Verification items for this drawing (mm, ordinates from the low corner). A direction names the side the tool comes from. Give positions to 0.01 mm unless a question says otherwise; leave off trailing zeros. Loops run counter-clockwise (first coordinate to the right, second up) from the corner with the lowest first, then second, coordinate; pieces in that order, holes last. Notation, with made-up numbers: (53, 64.25) -> (62, 64.25) arc R24 cw to (62, 81.25) -> close; hole circle Ø11 at (-22, 64). An arc over 180 degrees is marked (long way). Use one line per item in the form item = value. Start each with the question number.
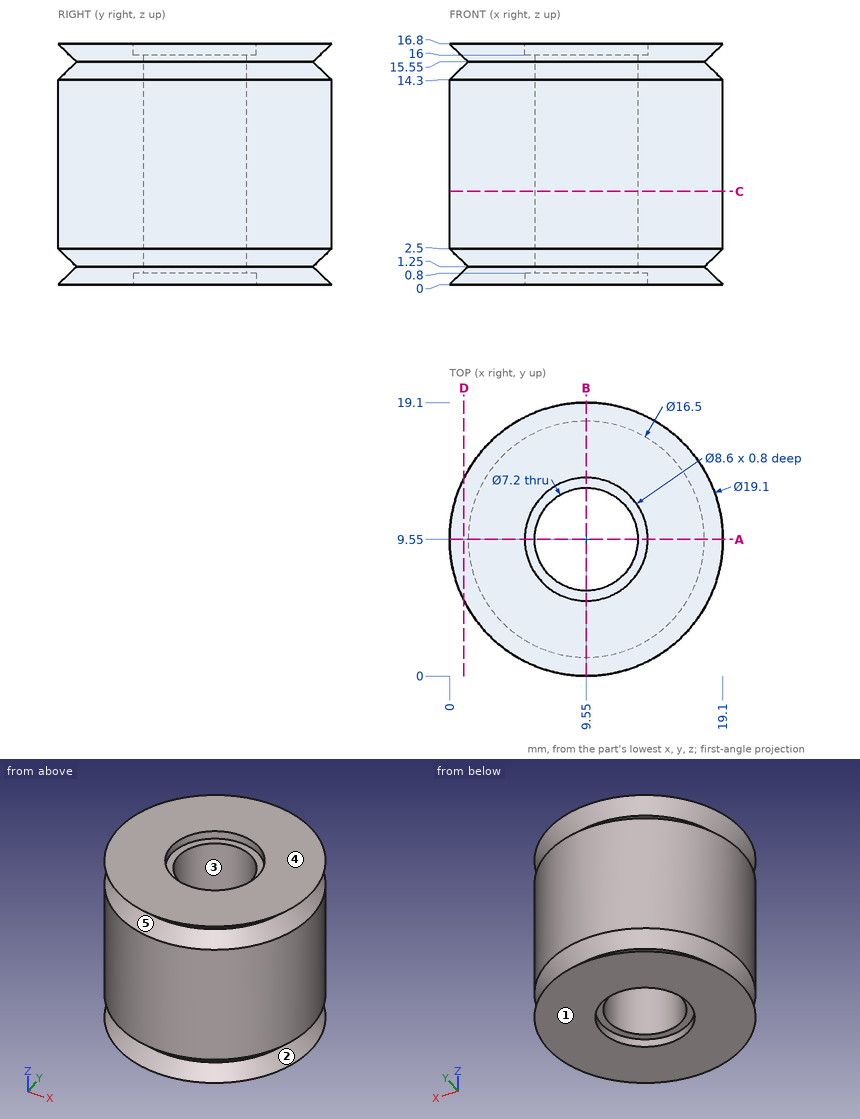
Item 1: Tool access check on the marked faces 4 and 5. Record the directions out of +Z, -Z, +X, -X, +Y, -Y that give a thin tool (end or side, any length) a straight path to the whole face; none if there is none.
Item 2: Sectioned sample at C-C, the plane z = 6.5. Enter the section's corners in (x, y).
Item 3: Draft check along Z on the marked faces 1, 2 and 3. Enter one of: +Z half, -Z half, draft (parallel to the pull), parting line (faces both ways), or undercut.
Item 4: Sectioned sample at D-D, the plane x = 1. State how many separate pieces and enclosed holes the cut face has, and give its area (3 significant figures).
Item 5: Sectioned sample at A-A, the plane y = 9.55. Enter the section's corners in (x, z).
Item 6: Material ranges on line 1 (Y direction, x = 9.75, z = 9); line 2 (Z direction, x = 2.5, y = 15.75); line 3 (Y direction, x = 11.5, z = 4.5), recorded low to high.
Item 7: Gauge pin test, flat ends, axial feed: pin 1 Ø4 at (y, z) = (13.5, 4) entering from +X; pin 2 Ø7.5 at (x, y) = (9.55, 9.55) entering from -Z; pin 3 Ø2 at (y, z) = (14.5, 14.5) entering from +X. Record the tip position at first contact, or that the pin passes through.
Outcome:
q1.face_4 = +Z, +X, -X, +Y, -Y
q1.face_5 = none
q2.outline = circle Ø19.1 at (9.55, 9.55); hole circle Ø7.2 at (9.55, 9.55)
q3.face_1 = -Z half
q3.face_2 = undercut
q3.face_3 = draft
q4.separate_pieces = 3
q4.enclosed_holes = 0
q4.area = 122 mm^2
q5.outline = (0, 0) -> (5.25, 0) -> (5.25, 0.8) -> (5.95, 0.8) -> (5.95, 16) -> (5.25, 16) -> (5.25, 16.8) -> (0, 16.8) -> (1.3, 15.55) -> (0, 14.3) -> (0, 2.5) -> (1.3, 1.25) -> close; (13.15, 0.8) -> (13.85, 0.8) -> (13.85, 0) -> (19.1, 0) -> (17.8, 1.25) -> (19.1, 2.5) -> (19.1, 14.3) -> (17.8, 15.55) -> (19.1, 16.8) -> (13.85, 16.8) -> (13.85, 16) -> (13.15, 16) -> close
q6.line_1 = 0 to 5.96, 13.14 to 19.1
q6.line_2 = 0 to 0.16, 2.34 to 14.46, 16.64 to 16.8
q6.line_3 = 0.2 to 6.52, 12.58 to 18.9
q7.pin_1 = 18.9
q7.pin_2 = 0.8
q7.pin_3 = 18.24
